```python
from build123d import *

# Parameters (mm, degrees)
SKETCH1_W               = 6.35
SKETCH1_H               = 61.468
BOSS_EXTRUDE1_DEPTH     = 31.75
BOSS_EXTRUDE2_DEPTH     = 12.7
SKETCH7_R               = 6.35
SKETCH8_R               = 4.6355
CUT_EXTRUDE1_DEPTH      = 169.831490025
CUT_EXTRUDE2_DEPTH      = 166.258966546
CUT_EXTRUDE2_DEPTH_BACK = 166.258966546
SKETCH12_W              = 13.716
SKETCH12_H              = 12.7


with BuildPart() as part:
    # Sketch1 → Boss-Extrude1 (new, symmetric)
    with BuildSketch(Plane(origin=(0, 0, 0), x_dir=(0, 0, -1), z_dir=(1, 0, 0))):
        with Locations((-3.175, 30.734)):
            Rectangle(SKETCH1_W, SKETCH1_H)
    extrude(amount=BOSS_EXTRUDE1_DEPTH, both=True)

    # Sketch4 → Boss-Extrude2 (add)
    with BuildSketch(Plane(origin=(31.75, 0, 0), x_dir=(0, 0, -1), z_dir=(1, 0, 0))):
        Polygon((-6.35, 0), (140.97, 0), (122.101981581, 6.168018419), (-6.35, 6.168018419), align=None)
    boss_extrude2 = extrude(amount=-BOSS_EXTRUDE2_DEPTH)

    # Mirror1: Boss-Extrude2 across plane
    add(boss_extrude2.mirror(Plane(origin=(0, 0, 0), x_dir=(0, 0, 1), z_dir=(1, 0, 0))))

    # Sweep1: sweep along a curve in space
    with BuildLine() as sweep1_path:
        Line((31.75, 61.468, 0), (-31.75, 61.468, 0))
    # Sketch7 → Sweep1 (sweep)
    with BuildSketch(Plane(origin=(31.75, 0, 0), x_dir=(0, 0, -1), z_dir=(1, 0, 0))):
        with Locations((0, 61.468)):
            Circle(SKETCH7_R)
    sweep(path=sweep1_path.line)

    # Sketch8 → Cut-Extrude1 (cut, through all)
    with BuildSketch(Plane(origin=(31.75, 0, 0), x_dir=(0, 0, -1), z_dir=(1, 0, 0))):
        with Locations((0, 61.468)):
            Circle(SKETCH8_R)
    extrude(amount=-CUT_EXTRUDE1_DEPTH, mode=Mode.SUBTRACT)

    # Sketch12 → Cut-Extrude2 (cut, two sides: drawn at the far end of the back side and taken through both)
    with BuildSketch(Plane.XY.offset(6.35).offset(-CUT_EXTRUDE2_DEPTH_BACK)):
        with Locations((-24.892, 61.468)):
            Rectangle(SKETCH12_W, SKETCH12_H)
        with Locations((24.892, 61.468)):
            Rectangle(SKETCH12_W, SKETCH12_H)
        with Locations((0, 61.468)):
            Rectangle(SKETCH12_W, SKETCH12_H)
    extrude(amount=CUT_EXTRUDE2_DEPTH + CUT_EXTRUDE2_DEPTH_BACK, mode=Mode.SUBTRACT)


solid = part.part
```
Check sheet for the modelled part. Datum: model origin and axes. Units: mm. A direction names the side the tool comes from. Round coordinates to 2 decimals unless told otherwise and drop trailing zeros. Order: outer loops, then holes, each group sorted by start corner. A loop starts at its lowest first (then second) coordinate and runs counter-clockwise, first axis right, second up. Notation, with made-up numbers: (-7, -37.75) -> (4, -37.75) arc R15 cw to (4, -18.75) -> close; hole circle Ø11 at (33.5, 29). An arc over 180 degrees is marked (long way). One line per item, written item: value. Start each with the question number.
Q1. Gauge pin test, flat ends, axial feed: pin 1 Ø10 at (x, z) = (27, -42) entering from +Y; pin 2 Ø3 at (x, z) = (-3.5, 2.5) entering from +Y; pin 3 Ø4 at (x, z) = (16, -53) entering from -Y; pin 4 Ø10 at (y, z) = (63, 0) entering from +X. Record the tip position at first contact, or that the pin passes through.
Q2. Mould release check, pull along X, two halves, no side actions. Record for faces 6 (the face through (-12.524, 66.104, -4.34)), 7 (the face through (31.75, 5, -46)), 8 (the face through (6.858, 58.6, 4.1)): pulls with the +X half, pulls with the -X half, needs draft (parallel to the pull), parting line crosses it, or undercut.
Q3. Thickness scan on line 1 (Z direction, x = 25.5, y = 19); line 2 (Y direction, x = -24.5, z = -45.5). Record the ranges inside material, lowest first.
Q4. Cross-section at A-A (z = -103). Record the boundary of the cut face in (x, y), and give its area (3 significant figures).
Q5. Set-up check for faces 1 (the face through (18.034, 58.6, 4.1)), 2 (the face through (-12.37, 56.94, 1)), 3 (the face through (-19.05, 3, -69)), 4 (the face through (-6.858, 58.6, 4.1)), 5 (the face through (22, 0, -66)): record each of +Z, -Z, +X, -X, +Y, -Y from which the full face is reachable in a straight line by a thin tool's end or side.
Q6. Cross-section at C-C (y = 10). Record the boundary of the cut face in (x, z), and give its area (3 significant figures).
Q7. Cross-section at B-B (x = 24.5). Record the boundary of the cut face in (y, z).
Completed:
1. pin 1: stops at y = 6.17
1. pin 2: stops at y = 55.12
1. pin 3: passes through
1. pin 4: stops at x = 18.03
2. face 6: needs draft
2. face 7: pulls with the +X half
2. face 8: undercut
3. line 1: z = 0 to 6.35
3. line 2: y = 0 to 6.17
4. outline: (-31.75, 0) -> (-19.05, 0) -> (-19.05, 6.17) -> (-31.75, 6.17) -> close; (19.05, 0) -> (31.75, 0) -> (31.75, 6.17) -> (19.05, 6.17) -> close
4. area: 157 mm²
5. face 1: +Z, -Z, +X, +Y
5. face 2: +X, -X
5. face 3: -Z, +Y, -Y
5. face 4: +Z, -Z, +Y
5. face 5: +Z, -Z, +X, -X, -Y
6. outline: (-31.75, 0) -> (31.75, 0) -> (31.75, 6.35) -> (-31.75, 6.35) -> close
6. area: 403 mm²
7. outline: (0, -140.97) -> (6.17, -122.1) -> (6.17, 0) -> (55.12, 0) -> (55.12, 6.35) -> (0, 6.35) -> close
